Source: CAD feature listing. Evaluate the final solid. Frame: model axes, mm. Face numbers are marked on the shaded views. A direction names the side the tool comes from. Round coordinates to 2 decimals unless told otherwise and drop trailing zeros. Order: outer loops, then holes, each group sorted by start corner. A loop starts at its lowest first (then second) coordinate and runs counter-clockwise, first axis right, second up. Notation, with made-up numbers: (7, 87) - (18, 87) arc R11 ccw to (18, 106) - close; hole circle Ø6 at (72.25, 61). An arc over 180 degrees is marked (long way). Return JSON: item names as keys, results as strings. Group by question number.
1) Section D-D, the plane z = -3. Return loops of the section in (x, y).
2) Section C-C, the plane y = 2.25. Return loops of the section in (x, z), plus the area to 3 significant figures.
3) Section A-A, the plane y = 29. Return loops of the section in (x, z).
4) Contact query for flat-ended pins moving along their axis: P1, Ø2, axis at x = 16, y = 15, coming from the +Z side; P2, Ø3, axis at y = 5, z = -4, coming from the +X side; P3, Ø5, axis at x = 21, y = 18, coming from the -Z side; P4, Ø1.1, axis at x = 24, y = 5, coming from the -Z side. Output: stop coordinate, or through.
5) Ray query, line 1 (Y direction, x = 4.95, z = 0.65); line 2 (Z direction, x = 13.5, y = 22); line 3 (X direction, y = 12, z = 1.5). Return the intervals inside material, ascending. Write a range as from..to.
6) Mould query, pull axis X, two halves, no side actions, for the marked faces 6, 7 and 8. Classes: pulls with the +X half, pulls with the -X half, needs draft (parallel to the pull), parting line crosses it, or undercut.
7) Section B-B, the plane x = 33.05. Return loops of the section in (y, z), plus the area to 3 significant figures.
8) Access query for the marked faces 1, 2, 3, 4 and 5. Directions: +Z, -Z, +X, -X, +Y, -Y. A direction counts if a zero-diameter tool reaches every point of the face in a straight line with its end or side. Return the directions, or none.
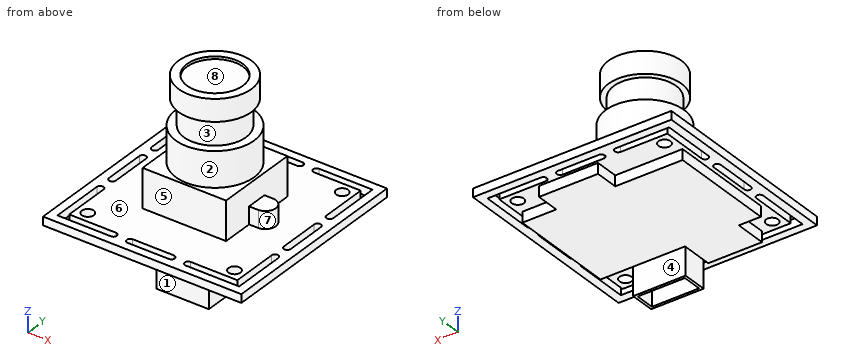
Autodesk Inventor part; units mm, degrees
ref_plane "YZ Plane" through (0, 0, 0) normal (1, 0, 0) x (0, 1, 0)
ref_plane "XZ Plane" through (0, 0, 0) normal (0, 1, 0) x (-1, 0, 0)
ref_plane "XY Plane" through (0, 0, 0) normal (0, 0, 1) x (1, 0, 0)
sketch "Sketch1" plane through (0, 0, 0) normal (0, 0, 1) x (1, 0, 0)
  line L0 (0, 0) -> (38, 0)
  line L1 (38, 0) -> (38, 38)
  line L2 (38, 38) -> (0, 38)
  line L3 (0, 38) -> (0, 0)
  line L4 (35.1, 35.1) -> (2.9, 35.1)
  line L5 (0, 38) -> (38, 0) construction
  line L6 (38, 38) -> (0, 0) construction
  line L7 (19, 0) -> (19, 38) construction
  line L8 (0, 19) -> (38, 19) construction
  arc A0 (11.85, 1.6) -> (11.85, 2.9) centre (11.85, 2.25) ccw
  arc A1 (15.05, 2.9) -> (15.05, 1.6) centre (15.05, 2.25) ccw
  arc A2 (22.95, 1.6) -> (22.95, 2.9) centre (22.95, 2.25) ccw
  arc A3 (26.15, 2.9) -> (26.15, 1.6) centre (26.15, 2.25) ccw
  line L9 (2.9, 2.9) -> (11.85, 2.9)
  line L10 (11.85, 1.6) -> (1.6, 1.6)
  line L11 (36.4, 1.6) -> (26.15, 1.6)
  line L12 (22.95, 1.6) -> (15.05, 1.6)
  line L13 (15.05, 2.9) -> (22.95, 2.9)
  line L14 (26.15, 2.9) -> (35.1, 2.9)
  arc A4 (35.1, 26.15) -> (36.4, 26.15) centre (35.75, 26.15) ccw
  line L15 (35.1, 15.05) -> (35.1, 22.95)
  arc A5 (36.4, 22.95) -> (35.1, 22.95) centre (35.75, 22.95) ccw
  line L16 (36.4, 22.95) -> (36.4, 15.05)
  line L17 (36.4, 11.85) -> (36.4, 1.6)
  arc A6 (36.4, 11.85) -> (35.1, 11.85) centre (35.75, 11.85) ccw
  arc A7 (35.1, 15.05) -> (36.4, 15.05) centre (35.75, 15.05) ccw
  line L18 (35.1, 26.15) -> (35.1, 35.1)
  line L19 (36.4, 36.4) -> (36.4, 26.15)
  line L20 (35.1, 2.9) -> (35.1, 11.85)
  arc A8 (11.85, 35.1) -> (11.85, 36.4) centre (11.85, 35.75) ccw
  line L21 (22.95, 35.1) -> (15.05, 35.1)
  arc A9 (15.05, 36.4) -> (15.05, 35.1) centre (15.05, 35.75) ccw
  line L22 (15.05, 36.4) -> (22.95, 36.4)
  line L23 (26.15, 36.4) -> (36.4, 36.4)
  arc A10 (26.15, 36.4) -> (26.15, 35.1) centre (26.15, 35.75) ccw
  arc A11 (22.95, 35.1) -> (22.95, 36.4) centre (22.95, 35.75) ccw
  line L24 (11.85, 35.1) -> (2.9, 35.1)
  line L25 (1.6, 36.4) -> (11.85, 36.4)
  line L26 (35.1, 35.1) -> (26.15, 35.1)
  arc A12 (2.9, 11.85) -> (1.6, 11.85) centre (2.25, 11.85) ccw
  line L27 (2.9, 22.95) -> (2.9, 15.05)
  arc A13 (1.6, 15.05) -> (2.9, 15.05) centre (2.25, 15.05) ccw
  line L28 (1.6, 15.05) -> (1.6, 22.95)
  line L29 (1.6, 26.15) -> (1.6, 36.4)
  arc A14 (1.6, 26.15) -> (2.9, 26.15) centre (2.25, 26.15) ccw
  arc A15 (2.9, 22.95) -> (1.6, 22.95) centre (2.25, 22.95) ccw
  line L30 (2.9, 11.85) -> (2.9, 2.9)
  line L31 (1.6, 1.6) -> (1.6, 11.85)
  line L32 (2.9, 35.1) -> (2.9, 26.15)
  circle A16 centre (33.05, 4.95) radius 1.15
  line L33 (3.8, 34.2) -> (34.2, 34.2) construction
  line L34 (34.2, 34.2) -> (34.2, 3.8) construction
  line L35 (34.2, 3.8) -> (3.8, 3.8) construction
  line L36 (3.8, 3.8) -> (3.8, 34.2) construction
  circle A17 centre (4.95, 4.95) radius 1.15
  circle A18 centre (33.05, 33.05) radius 1.15
  circle A19 centre (4.95, 33.05) radius 1.15
  point P0 (23.6, 2.25)
  point P1 (14.4, 2.25)
  point P2 (25.5, 2.25)
  point P3 (12.5, 2.25)
  point P4 (19, 19)
  point P5 (35.75, 25.5)
  point P6 (35.75, 23.6)
  point P7 (35.75, 12.5)
  point P8 (35.75, 14.4)
  point P9 (12.5, 35.75)
  point P10 (14.4, 35.75)
  point P11 (25.5, 35.75)
  point P12 (23.6, 35.75)
  point P13 (2.25, 12.5)
  point P14 (2.25, 14.4)
  point P15 (2.25, 25.5)
  point P16 (2.25, 23.6)
  point P17 (2.9, 35.1)
  point P18 (26.15, 35.1)
  dimension "d0" = 38
  dimension "d1" = 38
  dimension "d4" = 9.2
  dimension "d5" = 13
  dimension "d8" = 360
  dimension "d10" = 2.3
  dimension "d11" = 0.9
extrude "Extrusion1" add sketch "Sketch1" along normal blind 1.6
sketch "Sketch2" plane through (0, 0, 1.6) normal (0, 0, 1) x (1, 0, 0)
  line L0 (11, 27) -> (27, 27)
  line L1 (27, 27) -> (27, 11)
  line L2 (27, 11) -> (11, 11)
  line L3 (11, 11) -> (11, 27)
  line L4 (38, 38) -> (0, 38) construction
  line L5 (19, 38) -> (19, 0) construction
  line L6 (0, 0) -> (38, 0) construction
  line L7 (38, 0) -> (38, 38) construction
  line L8 (38, 19) -> (0, 19) construction
  line L9 (0, 38) -> (0, 0) construction
  dimension "d14" = 16
  dimension "d15" = 16
extrude "Extrusion2" add sketch "Sketch2" along normal blind 7.4
sketch "Sketch3" plane through (0, 0, 1.6) normal (0, 0, 1) x (1, 0, 0)
  line L0 (38, 38) -> (0, 38) construction
  line L1 (19, 38) -> (19, 0) construction
  line L2 (0, 0) -> (38, 0) construction
  line L3 (27, 11) -> (27, 27)
  line L4 (27, 21) -> (28.7765, 21)
  line L5 (28.7765, 17) -> (27, 17)
  line L6 (27, 17) -> (27, 21)
  arc A0 (28.7765, 17) -> (28.7765, 21) centre (28.6457, 19) ccw
  line L7 (0, 38) -> (0, 0) construction
  line L8 (0, 19) -> (38, 19) construction
  line L9 (38, 0) -> (38, 38) construction
  line L10 (11, 11) -> (11, 27)
  line L11 (11, 21) -> (9.2235, 21)
  line L12 (9.2235, 17) -> (11, 17)
  line L13 (11, 17) -> (11, 21)
  arc A1 (9.2235, 21) -> (9.2235, 17) centre (9.3543, 19) ccw
  line L14 (38, 19) -> (0, 19) construction
  point P0 (27.8883, 21)
  point P1 (10.1117, 21)
  point P2 (30.65, 19)
  point P3 (7.35, 19)
  dimension "d18" = 4
  dimension "d19" = 23.3
extrude "Extrusion3" add sketch "Sketch3" along normal blind 3.3
sketch "Sketch4" plane through (0, 0, 9) normal (0, 0, 1) x (1, 0, 0)
  line L0 (27, 27) -> (11, 27) construction
  line L1 (19, 27) -> (19, 11) construction
  line L2 (27, 11) -> (11, 11) construction
  line L3 (27, 11) -> (27, 27) construction
  line L4 (27, 19) -> (11, 19) construction
  line L5 (11, 27) -> (11, 11) construction
  circle A0 centre (19, 19) radius 7.5
  point P0 (0, 0)
  dimension "d22" = 15
extrude "Extrusion4" add sketch "Sketch4" along normal blind 6.7
sketch "Sketch5" plane through (19, 19, 15.7) normal (0, 0, 1) x (1, 0, 0)
  circle A0 centre (0, 0) radius 7.5
  circle A1 centre (0, 0) radius 5.925
  point P0 (-19, -19)
  dimension "d25" = 11.85
extrude "Extrusion5" add sketch "Sketch5" along normal blind 5 contours A1
sketch "Sketch6" plane through (19, 19, 20.7) normal (0, 0, 1) x (1, 0, 0)
  circle A0 centre (0, 0) radius 5.925
  circle A1 centre (0, 0) radius 6.975
  point P0 (-19, -19)
  dimension "d28" = 13.95
extrude "Extrusion6" add sketch "Sketch6" along normal blind 4.2 contours A0 | A1
sketch "Sketch7" plane through (19, 19, 24.9) normal (0, 0, 1) x (1, 0, 0)
  circle A0 centre (0, 0) radius 6.975
  circle A1 centre (0, 0) radius 5.35
  point P0 (-19, -19)
  dimension "d31" = 10.7
extrude "Extrusion7" cut sketch "Sketch7" against normal blind 0.5 contours A1
sketch "Sketch8" plane through (0, 0, 0) normal (0, 0, -1) x (-1, 0, 0)
  line L0 (-29.2, 8.2) -> (-19.15, 8.2)
  line L1 (-19.15, 8.2) -> (-19.15, 3.5)
  line L2 (-19.15, 3.5) -> (-29.2, 3.5)
  line L3 (-29.2, 3.5) -> (-29.2, 8.2)
  line L4 (-38, 0) -> (-38, 38)
  line L5 (0, 0) -> (-38, 0)
  dimension "d34" = 10.05
  dimension "d35" = 4.7
  dimension "d36" = 8.8
  dimension "d37" = 3.5
extrude "Extrusion8" add sketch "Sketch8" along normal blind 6.2
sketch "Sketch9" plane through (0, 0, -6.2) normal (0, 0, -1) x (-1, 0, 0)
  line L0 (-29.2, 3.5) -> (-19.15, 3.5)
  line L1 (-19.15, 3.5) -> (-19.15, 8.2)
  line L2 (-19.15, 8.2) -> (-29.2, 8.2)
  line L3 (-29.2, 8.2) -> (-29.2, 3.5)
  line L4 (-28.7, 7.7) -> (-19.65, 7.7)
  line L5 (-19.65, 7.7) -> (-19.65, 4)
  line L6 (-19.65, 4) -> (-28.7, 4)
  line L7 (-28.7, 4) -> (-28.7, 7.7)
  point P0 (0, 0)
  dimension "d40" = 0.5
extrude "Extrusion9" cut sketch "Sketch9" against normal blind 4.8 contours L4 L5 L6 L7
sketch "Sketch10" plane through (0, 0, 0) normal (0, 0, -1) x (-1, 0, 0)
  line L0 (-34.35, 30.1061) -> (-3.65, 30.1061)
  line L1 (-3.65, 30.1061) -> (-3.65, 9.7)
  line L2 (-3.65, 9.7) -> (-34.35, 9.7)
  line L3 (-34.35, 9.7) -> (-34.35, 30.1061)
  line L4 (-2.9, 22.95) -> (-2.9, 15.05)
  line L5 (-35.1, 15.05) -> (-35.1, 22.95)
  line L6 (-35.1, 35.1) -> (-26.15, 35.1)
  line L7 (-27.85, 30.1061) -> (-16.55, 30.1061)
  line L8 (-16.55, 30.1061) -> (-16.55, 34.6)
  line L9 (-16.55, 34.6) -> (-27.85, 34.6)
  line L10 (-27.85, 34.6) -> (-27.85, 30.1061)
  line L11 (-18.15, 9.7) -> (-7.85, 9.7)
  line L12 (-7.85, 9.7) -> (-7.85, 3.65)
  line L13 (-7.85, 3.65) -> (-18.15, 3.65)
  line L14 (-18.15, 3.65) -> (-18.15, 9.7)
  line L15 (-19.15, 8.2) -> (-29.2, 8.2)
  line L16 (-19.15, 3.5) -> (-19.15, 8.2)
  line L17 (-15.05, 2.9) -> (-22.95, 2.9)
  line L18 (-22.95, 35.1) -> (-15.05, 35.1)
  line L19 (-38, 0) -> (-38, 38)
  point P0 (0, 0)
  dimension "d43" = 0.75
  dimension "d44" = 0.75
  dimension "d45" = 4.9939
  dimension "d46" = 1.5
  dimension "d47" = 1
  dimension "d48" = 0.75
  dimension "d49" = 10.3
  dimension "d50" = 0.5
  dimension "d51" = 10.15
  dimension "d52" = 11.3
extrude "Extrusion10" add sketch "Sketch10" along normal blind 2
properties part number "Camera2"
Geometry check:
{
 "1": {"outline": "(19.15, 3.5) - (29.2, 3.5) - (29.2, 8.2) - (19.15, 8.2) - close; hole (19.65, 4) - (28.7, 4) - (28.7, 7.7) - (19.65, 7.7) - close"},
 "2": {"outline": "(0, 0) - (1.6, 0) - (1.6, 1.6) - (0, 1.6) - close; (12.5, 0) - (14.4, 0) - (14.4, 1.6) - (12.5, 1.6) - close; (23.6, 0) - (25.5, 0) - (25.5, 1.6) - (23.6, 1.6) - close; (36.4, 0) - (38, 0) - (38, 1.6) - (36.4, 1.6) - close", "area": "11.2 mm2"},
 "3": {"outline": "(0, 0) - (1.6, 0) - (1.6, 1.6) - (0, 1.6) - close; (2.9, 0) - (3.65, 0) - (3.65, -2) - (34.35, -2) - (34.35, 0) - (35.1, 0) - (35.1, 1.6) - (2.9, 1.6) - close; (36.4, 0) - (38, 0) - (38, 1.6) - (36.4, 1.6) - close"},
 "4": {"P1": "z = 24.9", "P2": "x = 29.2", "P3": "z = -2", "P4": "z = -1.4"},
 "5": {"line 1": "0..1.6, 2.9..3.8, 6.1..31.9, 34.2..35.1, 36.4..38", "line 2": "-2..15.7, 20.7..24.9", "line 3": "0..1.62, 2.88..35.12, 36.38..38"},
 "6": {"face 6": "needs draft", "face 7": "pulls with the +X half", "face 8": "undercut"},
 "7": {"outline": "(0, 0) - (1.6, 0) - (1.6, 1.6) - (0, 1.6) - close; (2.9, 0) - (3.8, 0) - (3.8, 1.6) - (2.9, 1.6) - close; (6.1, 0) - (9.7, 0) - (9.7, -2) - (30.11, -2) - (30.11, 0) - (31.9, 0) - (31.9, 1.6) - (6.1, 1.6) - close; (34.2, 0) - (35.1, 0) - (35.1, 1.6) - (34.2, 1.6) - close; (36.4, 0) - (38, 0) - (38, 1.6) - (36.4, 1.6) - close", "area": "90.1 mm2"},
 "8": {"face 1": "-Z, +X, -X, -Y", "face 2": "+Z", "face 3": "none", "face 4": "-Z, +X", "face 5": "+Z, +X, -X, -Y"}
}
